Build history of the part. All positions in model axes, mm. A direction names the side the tool comes from. Coordinates: 2 decimals unless noted, no trailing zeros. Order: outer loops, then holes, each group sorted by start corner. A loop starts at its lowest first (then second) coordinate and runs counter-clockwise, first axis right, second up. Notation, with made-up numbers: (25, 64) -> (30, 64) arc R12 ccw to (30, 82) -> close; hole circle Ø11 at (83.5, 45). An arc over 180 degrees is marked (long way). Write each question's results on one line, items separated by ' | '.
from build123d import *

# Parameters (mm, degrees)
F0_W     = 36
F0_H     = 75
F1_DEPTH = 30
F2_T     = -3
F4_D     = 5


with BuildPart() as f1:
    # F0 (on Top) → F1 (new body)
    with BuildSketch(Plane.XY):
        with Locations((18, 37.5)):
            Rectangle(F0_W, F0_H)
    extrude(amount=F1_DEPTH)

    # F2
    f2_openings = [f1.faces().sort_by_distance(p)[0] for p in [
        (18, 0, 15),
        (18, 37.5, 30),
        (18, 75, 15),
    ]]
    offset(amount=F2_T, openings=f2_openings)

    # F4 (through all)
    with Locations(Plane(origin=(0, 0, 0), x_dir=(1, 0, 0), z_dir=(0, 0, -1))):
        with Locations((17.4995128149, -20.8268326492), (16.5131200809, -56.3370103376)):
            Hole(F4_D / 2)


solid = f1.part
Item 1: Tool access for faces 1 (the flat face through (17.9, 75, 2.7)), 2 (the flat face through (18, 38, 3)): list every direction of +Z, -Z, +X, -X, +Y, -Y with a clear straight run to the whole face (end or side of a thin tool).
Answer:
face 1: +Z, -Z, +X, -X, +Y | face 2: +Z, +Y, -Y
Item 2: Pin check, flat tip, straight feed: pin 1 (3 mm diameter, centred on x = 18.5, y = 57, fed in from +Z). Stop position of the tip, or through.
Answer:
pin 1: stops at z = 3
Item 3: Pull direction X, two halves, no side cores. Call faces 3 (the flat face through (34, 38, 30)), 4 (the flat face through (33, 37, 16)), 5 (the flat face through (36, 37, 15)): released by +X, released by -X, zero draft, split by the parting line, or undercut.
Answer:
face 3: zero draft | face 4: undercut | face 5: released by +X
Item 4: Slice it at B-B, the plane y = 22. List the corners of the cut face in (x, z), and give its area (3 significant figures).
Answer:
outline: (0, 0) -> (15.29, 0) -> (15.29, 3) -> (3, 3) -> (3, 30) -> (0, 30) -> close; (19.71, 0) -> (36, 0) -> (36, 30) -> (33, 30) -> (33, 3) -> (19.71, 3) -> close | area: 257 mm^2
Item 5: Drill centre lines: line 1 (X direction, y = 62, z = 5.5); line 2 (Z direction, x = 28.5, y = 59.5). Where is each one in solid material? Low to high. Write a range as from..to.
Answer:
line 1: x = 0..3, 33..36 | line 2: z = 0..3
Item 6: Slice it at A-A, the plane z = 5.75. List the corners of the cut face in (x, y), and give its area (3 significant figures).
Answer:
outline: (0, 0) -> (3, 0) -> (3, 75) -> (0, 75) -> close; (33, 0) -> (36, 0) -> (36, 75) -> (33, 75) -> close | area: 450 mm^2
Item 7: Slice it at C-C, the plane x = 12. List the corners of the cut face in (y, z), and give its area (3 significant figures).
Answer:
outline: (0, 0) -> (75, 0) -> (75, 3) -> (0, 3) -> close | area: 225 mm^2
